from build123d import *

# Parameters (mm, degrees)
SKETCH3_W           = 76.2
SKETCH3_H           = 25.4
SKETCH3_W_2         = 69.85
SKETCH3_H_2         = 19.05
BOSS_EXTRUDE1_DEPTH = 457.2
SKETCH4_W           = 14.2875
SKETCH4_H           = 25.4
CUT_EXTRUDE1_DEPTH  = 464.680461094


with BuildPart() as part:
    # Sketch3 → Boss-Extrude1 (new, symmetric)
    with BuildSketch(Plane.XY):
        Rectangle(SKETCH3_W, SKETCH3_H)
        Rectangle(SKETCH3_W_2, SKETCH3_H_2, mode=Mode.SUBTRACT)
    extrude(amount=BOSS_EXTRUDE1_DEPTH, both=True)

    # Sketch4 → Cut-Extrude1 (cut, through all)
    with BuildSketch(Plane(origin=(38.1, 0, 0), x_dir=(0, 0, -1), z_dir=(1, 0, 0))):
        with Locations((-450.05625, 0)):
            Rectangle(SKETCH4_W, SKETCH4_H)
        Polygon((-442.9125, -12.7), (-415.13125, 12.7), (-442.9125, 12.7), align=None)
        with Locations((450.05625, 0)):
            Rectangle(SKETCH4_W, SKETCH4_H)
        Polygon((442.9125, -12.7), (442.9125, 12.7), (415.13125, 12.7), align=None)
    extrude(amount=-CUT_EXTRUDE1_DEPTH, mode=Mode.SUBTRACT)


solid = part.part
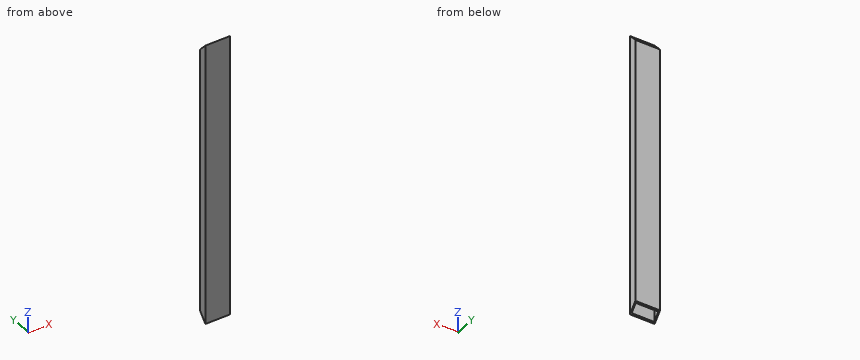
Verification items for the finished model (mm, model axes). Give positions to 0.01 mm unless a question says otherwise; leave off trailing zeros. Write each loop counter-clockwise with the first axis right and the second up, starting at its lowest first coordinate (ties: lowest second). Pieces come first, ordered by that corner, then holes. Notation, with made-up numbers: M 87,-12.75 L 94,-12.75 A32 ccw 94,21.25 Z; hole C 3,48 d6. An arc over 180 degrees is marked long. Put each result on its own line as item: value. Start each with the question number.
1. Section check B-B (x = -6.5). Record the cut outline in (y, z) (1 decimal).
2. Section check C-C (y = -0.75). Record the cut outline in (x, z) (3 decimals), and give its area (3 significant figures).
3. Scan lines: line 1 along X through (y, z) = (3.5, -303) (3 decimals); line 2 along Y through (x, z) = (19.5, -186.5) (3 decimals); line 3 along Z through (x, y) = (-32, -9.75). Record each from-to range of solid material in increasing order. Write a range as [from, to].
4. Section check A-A (z = -179). Record the cut outline in (x, y) (3 decimals).
Answer list:
1. outline: M -12.7,-442.9 L -9.5,-439.4 L -9.5,439.4 L -12.7,442.9 Z; M 9.5,-418.6 L 12.7,-415.1 L 12.7,415.1 L 9.5,418.6 Z
2. outline: M -38.1,-429.842 L -34.925,-429.842 L -34.925,429.842 L -38.1,429.842 Z; M 34.925,-429.842 L 38.1,-429.842 L 38.1,429.842 L 34.925,429.842 Z
2. area: 5,460 mm2
3. line 1: [-38.1, -34.925], [34.925, 38.1]
3. line 2: [-12.7, -9.525], [9.525, 12.7]
3. line 3: [-439.69, 439.69]
4. outline: M -38.1,-12.7 L 38.1,-12.7 L 38.1,12.7 L -38.1,12.7 Z; hole M -34.925,-9.525 L 34.925,-9.525 L 34.925,9.525 L -34.925,9.525 Z
